Work out the finished part from the listing and answer in its coordinate system (mm). Face numbers are marked on the shaded views. A direction names the side the tool comes from. Give positions to 0.01 mm unless a question says otherwise; leave off trailing zeros. Write each loop counter-clockwise with the first axis right and the second up, starting at its lowest first coordinate (ties: lowest second). Pieces come first, ordered by that corner, then holes. Notation, with made-up numbers: (-5, 79.25) -> (16, 79.25) arc R14 ccw to (16, 86.25) -> close; hole circle Ø9 at (69, 56.25). An arc over 180 degrees is marked (long way). Use a Markdown table: item, result. Add a question column.
Q1. For a pull along X with two mould halves and no side action, classify the marked faces 3, 4, 5 and 6 as pulls with the +X half, pulls with the -X half, needs draft (parallel to the pull), parting line crosses it, or undercut.
Q2. Section C-C, the plane z = 119.5 is taken. Give the vertices of the cut face in (x, y), plus the area to 3 significant figures.
Q3. Section A-A, the plane y = -12.7 is taken. State how many separate pieces and enclosed holes the cut face has, plus the area to 3 significant figures.
Q4. Each of these flat-tipped pins is pushed along its axis until it touches: pin 1 Ø3 at (y, z) = (-5.5, 175.5) entering from +X; pin 2 Ø2 at (y, z) = (-6.5, 53.5) entering from +X; pin 3 Ø0.5 at (y, z) = (-20.5, 54) entering from +X; pin 4 Ø13 at (x, z) = (0, 0) entering from +Y. Where does it stop, or does it pass through?
Q5. Consider line 1 (Y direction, x = -3, z = 53); line 2 (Z direction, x = -6, y = -13.5); line 3 (Z direction, x = 3, y = -19.5). Determine where each line is inside the solid, lowest interval first.
Q6. For the marked faces 1 and 2, determine the directions among +Z, -Z, +X, -X, +Y, -Y from which every point of the face is accessible in a straight line to the end or side of a thin tool.
from build123d import *

# Parameters (mm, degrees)
F0_R     = 10.795
F1_DEPTH = 25.4
F2_R     = 2.286
F3_R     = 3.556
F4_R     = 6.35
F5_R     = 2.5527
F6_DEPTH = 12.7


with BuildPart() as f1:
    # F0 (on Front) → F1 (new body)
    with BuildSketch(Plane.XZ):
        with BuildLine():
            Line((-14.2875, 200.66), (-14.2875, 0))
            ThreePointArc((-14.2875, 0), (12.600391, -6.735192), (-7.9375, 11.879762))
            Line((-7.9375, 11.879762), (-7.9375, 43.18))
            Line((-7.9375, 43.18), (16.9545, 43.18))
            Line((16.9545, 43.18), (16.9545, 49.53))
            Line((16.9545, 49.53), (-1.5875, 49.53))
            Line((-1.5875, 49.53), (-1.5875, 57.15))
            Line((-1.5875, 57.15), (-7.9375, 57.15))
            Line((-7.9375, 57.15), (-7.9375, 194.31))
            Line((-7.9375, 194.31), (17.4625, 194.31))
            Line((17.4625, 194.31), (17.4625, 184.785))
            Line((17.4625, 184.785), (23.8125, 184.785))
            Line((23.8125, 184.785), (23.8125, 200.66))
            Line((23.8125, 200.66), (-14.2875, 200.66))
        make_face()
        Circle(F0_R, mode=Mode.SUBTRACT)
    extrude(amount=F1_DEPTH)

    # F2
    f2_edges = [f1.edges().sort_by_distance(p)[0] for p in [
        (16.9545, -12.7, 43.18),
        (16.9545, -12.7, 49.53),
        (23.8125, -12.7, 184.785),
        (17.4625, -12.7, 184.785),
        (-1.5875, -12.7, 57.15),
    ]]
    fillet(f2_edges, radius=F2_R)

    # F3
    f3_edges = [f1.edges().sort_by_distance(p)[0] for p in [
        (17.4625, -12.7, 194.31),
        (-7.9375, -12.7, 194.31),
        (-7.9375, -12.7, 57.15),
        (-1.5875, -12.7, 49.53),
    ]]
    fillet(f3_edges, radius=F3_R)

    # F4
    f4_edges = [f1.edges().sort_by_distance(p)[0] for p in [
        (-7.9375, -12.7, 43.18),
        (23.8125, -12.7, 200.66),
        (-14.2875, -12.7, 200.66),
        (-7.9375, -12.7, 11.879762),
    ]]
    fillet(f4_edges, radius=F4_R)

    # F5 (on face) → F6 (cut, symmetric)
    with BuildSketch(Plane.YZ.offset(-7.9375)):
        with Locations((-12.7, 53.34)):
            Circle(F5_R)
    extrude(amount=F6_DEPTH, both=True, mode=Mode.SUBTRACT)


solid = f1.part
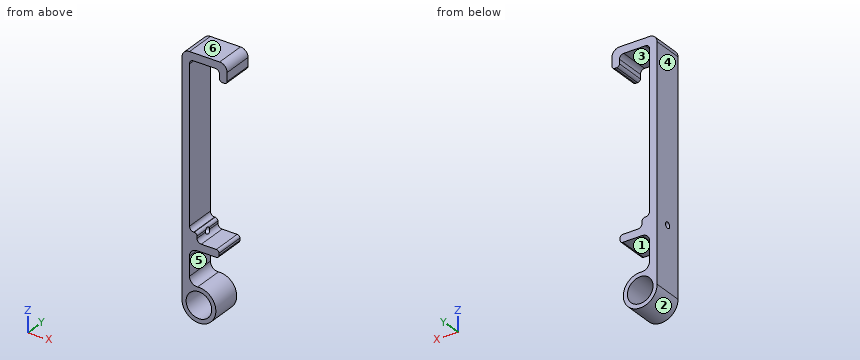
Result set:
| question | item | result |
|---|---|---|
| 1 | face 3 | undercut |
| 1 | face 4 | pulls with the -X half |
| 1 | face 5 | pulls with the +X half |
| 1 | face 6 | needs draft |
| 2 | outline | (-14.29, -25.4) -> (-7.94, -25.4) -> (-7.94, 0) -> (-14.29, 0) -> close |
| 2 | area | 161 mm2 |
| 3 | separate pieces | 2 |
| 3 | enclosed holes | 1 |
| 3 | area | 1,910 mm2 |
| 4 | pin 1 | stops at x = -7.94 |
| 4 | pin 2 | stops at x = -1.54 |
| 4 | pin 3 | stops at x = -1.59 |
| 4 | pin 4 | passes through |
| 5 | line 1 | y = -25.4 to -15.23, -10.17 to 0 |
| 5 | line 2 | z = -12.97 to -8.97, 8.97 to 16.01, 41.4 to 50.92, 55.76 to 57.54, 193.92 to 200.66 |
| 5 | line 3 | z = -13.97 to -10.37, 10.37 to 13.97, 43.18 to 49.53, 194.31 to 200.66 |
| 6 | face 1 | +X, +Y, -Y |
| 6 | face 2 | +Y, -Y |
